Autodesk Inventor part; units mm, degrees
ref_plane "YZ Plane" through (0, 0, 0) normal (1, 0, 0) x (0, 1, 0)
ref_plane "XZ Plane" through (0, 0, 0) normal (0, 1, 0) x (-1, 0, 0)
ref_plane "XY Plane" through (0, 0, 0) normal (0, 0, 1) x (1, 0, 0)
sketch "スケッチ1" plane through (0, 0, 0) normal (0, 0, 1) x (1, 0, 0)
  circle A0 centre (0, 0) radius 1.5
  dimension "d0" = 3
extrude "押し出し1" add sketch "スケッチ1" along normal blind 6
sketch "スケッチ2" plane through (0, 0, 6) normal (0, 0, 1) x (1, 0, 0)
  circle A0 centre (0, 0) radius 1.5
  circle A1 centre (0, 0) radius 3
  dimension "d3" = 6
extrude "押し出し2" add sketch "スケッチ2" along normal blind 1.75 contours A0 | A1
thread "ねじ1"
chamfer "面取り1" distance 1.5 angle 45 1 edges at (-3, 0, 6)
sketch "スケッチ4" plane through (0, 0, 0) normal (0, 0, -1) x (-1, 0, 0)
  circle A0 centre (0, 0) radius 1.5
extrude "押し出し4" add sketch "スケッチ4" along normal blind 4
sketch "スケッチ5" plane through (0, 0, -4) normal (0, 0, -1) x (-1, 0, 0)
  circle A0 centre (0, 0) radius 1.5
extrude "押し出し5" cut sketch "スケッチ5" against normal blind 1.75
properties part number "SB　10mm皿ネジ" material "Steel, Mild"
Here's how the part is built. I have some questions about the finished solid (model axes, mm). Round coordinates to 2 decimals unless told otherwise and drop trailing zeros. Loops run counter-clockwise (first coordinate to the right, second up) from the corner with the lowest first, then second, coordinate; pieces in that order, holes last. Notation, with made-up numbers: (-34, 88) -> (-19, 88) arc R9 ccw to (-19, 101) -> close; hole circle Ø11 at (3, 71). An arc over 180 degrees is marked (long way). Answer as CSV lines item,"result". Start each with the question number.
1. Imagine slicing it at C-C on z = 5.5. Write out the boundary of the cut face in (x, y).
2. I'm going to push flat-ended pins straight in: P1, Ø1.5, axis at x = 1.5, z = 4.5, coming from the +Y side; P2, Ø2, axis at x = 1.5, z = 2.5, coming from the -Y side. Where does each tip first touch, or does it pass through?
3. Imagine slicing it at D-D on z = 6.75. Write out the boundary of the cut face in (x, y).
4. I need wall thicknesses on probe 1 along Y at (x, z) = (0.1, 3.5); probe 2 along Z at (x, y) = (0.7, -1.85); probe 3 along Z at (x, y) = (2.3, 1.55). Which ranges of each line are inside material? Lowest first, please. Write a range as from..to.
Solution:
1,outline,"circle Ø3 at (0, 0)"
2,P1,"y = 1.3"
2,P2,"y = -1.41"
3,outline,"circle Ø4.5 at (0, 0)"
4,probe 1,"-1.5..1.5"
4,probe 2,"6.48..7.75"
4,probe 3,"7.27..7.75"
